from build123d import *

# Parameters (mm, degrees)
SKETCH6_R           = 2.6
SKETCH6_R_2         = 3.55
BOSS_EXTRUDE2_DEPTH = 1.5


with BuildPart() as part:
    # Sketch6 → Boss-Extrude2 (new body)
    with BuildSketch(Plane.XY):
        with BuildLine():
            Line((90, 120), (10.125875384, 120))
            ThreePointArc((10.125875384, 120), (3.017939526, 117.160075149), (0, 110.125875384))
            Line((0, 110.125875384), (0, 10))
            ThreePointArc((0, 10), (2.928932188, 2.928932188), (10, 0))
            Line((10, 0), (91.314001846, 0))
            ThreePointArc((91.314001846, 0), (96.901124962, 2.644656697), (99.896074117, 8.052099098))
            Line((99.896074117, 8.052099098), (99.896074117, 111.437955866))
            ThreePointArc((99.896074117, 111.437955866), (96.542951984, 117.562392434), (90, 120))
        make_face()
        with Locations((50, 17.7)):
            Circle(SKETCH6_R, mode=Mode.SUBTRACT)
        with Locations((17.7, 17.7)):
            Circle(SKETCH6_R_2, mode=Mode.SUBTRACT)
        with Locations((75.25, 17.7)):
            Circle(SKETCH6_R, mode=Mode.SUBTRACT)
        with Locations((40, 17.7)):
            Circle(SKETCH6_R, mode=Mode.SUBTRACT)
        with Locations((60, 90)):
            Circle(SKETCH6_R, mode=Mode.SUBTRACT)
        with Locations((40, 90)):
            Circle(SKETCH6_R, mode=Mode.SUBTRACT)
        with Locations((60, 102.3)):
            Circle(SKETCH6_R, mode=Mode.SUBTRACT)
        with Locations((10, 50)):
            Circle(SKETCH6_R, mode=Mode.SUBTRACT)
        with Locations((70, 50)):
            Circle(SKETCH6_R, mode=Mode.SUBTRACT)
        with Locations((90, 70)):
            Circle(SKETCH6_R, mode=Mode.SUBTRACT)
        with Locations((30, 70)):
            Circle(SKETCH6_R, mode=Mode.SUBTRACT)
        with Locations((10, 70)):
            Circle(SKETCH6_R, mode=Mode.SUBTRACT)
        with Locations((17.7, 102.3)):
            Circle(SKETCH6_R_2, mode=Mode.SUBTRACT)
        with Locations((60, 30)):
            Circle(SKETCH6_R, mode=Mode.SUBTRACT)
        with Locations((85.25, 60)):
            Circle(SKETCH6_R, mode=Mode.SUBTRACT)
        with Locations((40, 60)):
            Circle(SKETCH6_R, mode=Mode.SUBTRACT)
        with Locations((60, 40)):
            Circle(SKETCH6_R, mode=Mode.SUBTRACT)
        with Locations((50, 102.3)):
            Circle(SKETCH6_R, mode=Mode.SUBTRACT)
        with Locations((50, 60)):
            Circle(SKETCH6_R, mode=Mode.SUBTRACT)
        with Locations((50, 70)):
            Circle(SKETCH6_R, mode=Mode.SUBTRACT)
        with Locations((50, 50)):
            Circle(SKETCH6_R, mode=Mode.SUBTRACT)
        with Locations((60, 60)):
            Circle(SKETCH6_R, mode=Mode.SUBTRACT)
        with Locations((17.7, 60)):
            Circle(SKETCH6_R_2, mode=Mode.SUBTRACT)
        with Locations((85.25, 102.3)):
            Circle(SKETCH6_R, mode=Mode.SUBTRACT)
        with Locations((40, 40)):
            Circle(SKETCH6_R, mode=Mode.SUBTRACT)
        with Locations((27.7, 102.3)):
            Circle(SKETCH6_R_2, mode=Mode.SUBTRACT)
        with Locations((40, 30)):
            Circle(SKETCH6_R, mode=Mode.SUBTRACT)
        with Locations((70, 70)):
            Circle(SKETCH6_R, mode=Mode.SUBTRACT)
        with Locations((90, 50)):
            Circle(SKETCH6_R, mode=Mode.SUBTRACT)
        with Locations((30, 50)):
            Circle(SKETCH6_R, mode=Mode.SUBTRACT)
        with Locations((75.25, 102.3)):
            Circle(SKETCH6_R, mode=Mode.SUBTRACT)
        with Locations((40, 102.3)):
            Circle(SKETCH6_R, mode=Mode.SUBTRACT)
        with Locations((40, 80)):
            Circle(SKETCH6_R, mode=Mode.SUBTRACT)
        with Locations((60, 80)):
            Circle(SKETCH6_R, mode=Mode.SUBTRACT)
        with Locations((60, 17.7)):
            Circle(SKETCH6_R, mode=Mode.SUBTRACT)
        with Locations((27.7, 17.7)):
            Circle(SKETCH6_R_2, mode=Mode.SUBTRACT)
        with Locations((85.25, 17.7)):
            Circle(SKETCH6_R, mode=Mode.SUBTRACT)
    extrude(amount=BOSS_EXTRUDE2_DEPTH)


solid = part.part
For this review, take the finished solid that the model builds, in its own axes (mm). Coordinates: 2 decimals unless noted, no trailing zeros. Order: outer loops, then holes, each group sorted by start corner. A loop starts at its lowest first (then second) coordinate and runs counter-clockwise, first axis right, second up. Notation, with made-up numbers: (49, 1.5) - (89, 1.5) arc R14 ccw to (89, 25.5) - close; hole circle Ø10 at (59, 55). An arc over 180 degrees is marked (long way). Answer as CSV lines item,"result". Start each with the question number.
1) To check wall thickness, follow line 1 along Y through (x, z) = (90, 1.25); line 2 along Y through (x, z) = (75.25, 0.6); line 3 along Y through (x, z) = (85, 0.8). State the ranges of each line that lie inside material, in increasing order. Write a range as [from, to].
2) Draft analysis for pull direction X (two halves, no side actions). For faces 1 (the cylindrical face through (47.4, 60.1, 0.7)), 2 (the cylindrical face through (39.662, 92.578, 0.74)), 3 (the cylindrical face through (96.618, 117.497, 0.74)), state which applies: +X half, -X half, draft (parallel to the pull), parting line (faces both ways), or undercut.
3) Add section D-D (x = 40). Count the separate pieces of the cut face and the enclosed holes in it, then the cut area to 3 significant figures.
4) Add section C-C (x = 70). State the section outline as (y, z) points.
5) Add section A-A (y = 60). State the section outline as (x, z) points, then the cut area to 3 significant figures.
6) Add section B-B (y = 90). State the section outline as (x, z) points.
Result:
1,line 1,"[0, 47.4], [52.6, 67.4], [72.6, 120]"
1,line 2,"[0, 15.1], [20.3, 99.7], [104.9, 120]"
1,line 3,"[0, 15.11], [20.29, 57.41], [62.59, 99.71], [104.89, 120]"
2,face 1,"undercut"
2,face 2,"undercut"
2,face 3,"+X half"
3,separate pieces,"8"
3,enclosed holes,"0"
3,area,"125 mm^2"
4,outline,"(0, 0) - (47.4, 0) - (47.4, 1.5) - (0, 1.5) - close; (52.6, 0) - (67.4, 0) - (67.4, 1.5) - (52.6, 1.5) - close; (72.6, 0) - (120, 0) - (120, 1.5) - (72.6, 1.5) - close"
5,outline,"(0, 0) - (14.15, 0) - (14.15, 1.5) - (0, 1.5) - close; (21.25, 0) - (37.4, 0) - (37.4, 1.5) - (21.25, 1.5) - close; (42.6, 0) - (47.4, 0) - (47.4, 1.5) - (42.6, 1.5) - close; (52.6, 0) - (57.4, 0) - (57.4, 1.5) - (52.6, 1.5) - close; (62.6, 0) - (82.65, 0) - (82.65, 1.5) - (62.6, 1.5) - close; (87.85, 0) - (99.9, 0) - (99.9, 1.5) - (87.85, 1.5) - close"
5,area,"108 mm^2"
6,outline,"(0, 0) - (37.4, 0) - (37.4, 1.5) - (0, 1.5) - close; (42.6, 0) - (57.4, 0) - (57.4, 1.5) - (42.6, 1.5) - close; (62.6, 0) - (99.9, 0) - (99.9, 1.5) - (62.6, 1.5) - close"
